```python
from build123d import *

# Parameters (mm, degrees)
SKETCH1_R           = 76
SKETCH1_R_2         = 27.051
SKETCH1_R_3         = 6.25
BOSS_EXTRUDE1_DEPTH = 7
SKETCH3_R           = 27.051
BOSS_EXTRUDE2_DEPTH = 5
SKETCH4_R           = 6.25
CUT_EXTRUDE1_DEPTH  = 10
FILLET1_R           = 5


with BuildPart() as part:
    # Sketch1 → Boss-Extrude1 (new body)
    with BuildSketch(Plane(origin=(0, 0, 0), x_dir=(1, 0, 0), z_dir=(0, 1, 0))):
        with Locations(Location((0, 0, 0), (0, 0, 270))):
            Circle(SKETCH1_R)
        with Locations(Location((0, 0, 0), (0, 0, 270))):
            Circle(SKETCH1_R_2, mode=Mode.SUBTRACT)
        with Locations(Location((0, 62.5, 0), (0, 0, 270))):
            Circle(SKETCH1_R_3, mode=Mode.SUBTRACT)
        with Locations(Location((62.5, 0, 0), (0, 0, 270))):
            Circle(SKETCH1_R_3, mode=Mode.SUBTRACT)
        with Locations(Location((0, -62.5, 0), (0, 0, 270))):
            Circle(SKETCH1_R_3, mode=Mode.SUBTRACT)
        with Locations(Location((-62.5, 0, 0), (0, 0, 270))):
            Circle(SKETCH1_R_3, mode=Mode.SUBTRACT)
    extrude(amount=BOSS_EXTRUDE1_DEPTH)

    # Sketch3 → Boss-Extrude2 (add)
    with BuildSketch(Plane.XZ):
        with Locations(Location((0, 0, 0), (0, 0, 270))):
            Circle(SKETCH3_R)
    extrude(amount=-BOSS_EXTRUDE2_DEPTH)

    # Sketch4 → Cut-Extrude1 (cut)
    with BuildSketch(Plane(origin=(0, 7, 0), x_dir=(1, 0, 0), z_dir=(0, 1, 0))):
        with BuildLine():
            Line((27.751246841, -43.661149418), (17.007161012, -32.917063589))
            ThreePointArc((17.007161012, -32.917063589), (15.274204293, -33.756114768), (13.5, -34.504008477))
            Line((13.5, -34.504008477), (13.5, -62.5))
            ThreePointArc((13.5, -62.5), (25.524772494, -58.625813335), (36.553123822, -52.463026398))
            Line((36.553123822, -52.463026398), (27.751246841, -43.661149418))
        make_face()
        with BuildLine():
            Line((62.5, -13.5), (34.504008477, -13.5))
            ThreePointArc((34.504008477, -13.5), (33.756114768, -15.274204293), (32.917063589, -17.007161012))
            Line((32.917063589, -17.007161012), (43.66114941, -27.751246833))
            Line((43.66114941, -27.751246833), (52.463026398, -36.553123822))
            ThreePointArc((52.463026398, -36.553123822), (58.625813335, -25.524772494), (62.5, -13.5))
        make_face()
        with BuildLine():
            ThreePointArc((-13.5, -34.504008477), (-15.274204293, -33.756114768), (-17.007161012, -32.917063589))
            Line((-17.007161012, -32.917063589), (-27.751246874, -43.66114945))
            Line((-27.751246874, -43.66114945), (-36.553123822, -52.463026398))
            ThreePointArc((-36.553123822, -52.463026398), (-25.524772494, -58.625813335), (-13.5, -62.5))
            Line((-13.5, -62.5), (-13.5, -34.504008477))
        make_face()
        with BuildLine():
            ThreePointArc((-32.917063589, -17.007161012), (-33.756114768, -15.274204293), (-34.504008477, -13.5))
            Line((-34.504008477, -13.5), (-62.5, -13.5))
            ThreePointArc((-62.5, -13.5), (-58.625813335, -25.524772494), (-52.463026398, -36.553123822))
            Line((-52.463026398, -36.553123822), (-43.661149471, -27.751246894))
            Line((-43.661149471, -27.751246894), (-32.917063589, -17.007161012))
        make_face()
        with BuildLine():
            ThreePointArc((-34.504008477, 13.5), (-33.756114768, 15.274204293), (-32.917063589, 17.007161012))
            Line((-32.917063589, 17.007161012), (-43.66114943, 27.751246854))
            Line((-43.66114943, 27.751246854), (-52.463026398, 36.553123822))
            ThreePointArc((-52.463026398, 36.553123822), (-58.625813335, 25.524772494), (-62.5, 13.5))
            Line((-62.5, 13.5), (-34.504008477, 13.5))
        make_face()
        with BuildLine():
            ThreePointArc((-17.007161012, 32.917063589), (-15.274204293, 33.756114768), (-13.5, 34.504008477))
            Line((-13.5, 34.504008477), (-13.5, 62.5))
            ThreePointArc((-13.5, 62.5), (-25.524772494, 58.625813335), (-36.553123822, 52.463026398))
            Line((-36.553123822, 52.463026398), (-27.751246874, 43.66114945))
            Line((-27.751246874, 43.66114945), (-17.007161012, 32.917063589))
        make_face()
        with BuildLine():
            ThreePointArc((36.553123822, 52.463026398), (25.524772494, 58.625813335), (13.5, 62.5))
            Line((13.5, 62.5), (13.5, 34.504008477))
            ThreePointArc((13.5, 34.504008477), (15.274204293, 33.756114768), (17.007161012, 32.917063589))
            Line((17.007161012, 32.917063589), (27.751246906, 43.661149483))
            Line((27.751246906, 43.661149483), (36.553123822, 52.463026398))
        make_face()
        with BuildLine():
            ThreePointArc((62.5, 13.5), (58.625813335, 25.524772494), (52.463026398, 36.553123822))
            Line((52.463026398, 36.553123822), (43.66114945, 27.751246874))
            Line((43.66114945, 27.751246874), (32.917063589, 17.007161012))
            ThreePointArc((32.917063589, 17.007161012), (33.756114768, 15.274204293), (34.504008477, 13.5))
            Line((34.504008477, 13.5), (62.5, 13.5))
        make_face()
        with Locations(Location((35.706198162, 35.706198162, 0), (0, 0, 270))):
            Circle(SKETCH4_R)
        with Locations(Location((35.706198162, -35.706198162, 0), (0, 0, 270))):
            Circle(SKETCH4_R)
        with Locations(Location((-35.706198162, -35.706198162, 0), (0, 0, 270))):
            Circle(SKETCH4_R)
        with Locations(Location((-35.706198162, 35.706198162, 0), (0, 0, 270))):
            Circle(SKETCH4_R)
    extrude(amount=-CUT_EXTRUDE1_DEPTH, mode=Mode.SUBTRACT)

    # Fillet1
    # the kernel refuses this fillet: 5 mm, written as the material it adds along each edge
    with BuildSketch(Plane(origin=(34.504008477, 7, 13.5), x_dir=(1, 0, 0), z_dir=(0, -1, 0)), Plane(origin=(13.5, 7, -34.504008477), x_dir=(0, 0, -1), z_dir=(0, -1, 0)), Plane(origin=(-34.504008477, 7, -13.5), x_dir=(-1, 0, 0), z_dir=(0, -1, 0)), Plane(origin=(-13.5, 7, 34.504008477), x_dir=(0, 0, 1), z_dir=(0, -1, 0))) as fillet1_piece_1:
        with BuildLine():
            CenterArc((3.258891319, 5), FILLET1_R, 206.100178987, 63.899821013)
            ThreePointArc((-1.231239688, 2.800290124), (-0.586707725, 1.412857227), (0, 0))
            Line((0, 0), (3.258891319, 0))
        make_face()
    extrude(amount=7)
    with BuildSketch(Plane(origin=(62.5, 7, 13.5), x_dir=(-1, 0, 0), z_dir=(0, -1, 0))) as fillet1_piece_2:
        with BuildLine():
            CenterArc((6.537189081, -5), FILLET1_R, 90, 108.2926811)
            ThreePointArc((1.789861186, -6.569355874), (0.807426008, -3.308519097), (0, 0))
            Line((0, 0), (6.537189081, 0))
        make_face()
    extrude(amount=7)
    with BuildSketch(Plane(origin=(52.463026398, 7, 36.553123822), x_dir=(-0.7071067811865521, 0, -0.707106781186543), z_dir=(0, -1, 0)), Plane(origin=(-36.553123822, 7, 52.463026398), x_dir=(0.7071067811865515, 0, -0.7071067811865436), z_dir=(0, -1, 0))) as fillet1_piece_3:
        with BuildLine():
            CenterArc((6.286852353, 5), FILLET1_R, 163.996405934, 106.003594066)
            ThreePointArc((1.480630334, 6.378488268), (0.658610883, 3.208210045), (0, 0))
            Line((0, 0), (6.286852353, 0))
        make_face()
    extrude(amount=7)
    with BuildSketch(Plane(origin=(32.917063589, 7, 17.007161012), x_dir=(0.4193809358930841, 0, -0.907810349472532), z_dir=(0, -1, 0)), Plane(origin=(17.007161012, 7, -32.917063589), x_dir=(-0.9078103494725283, 0, -0.41938093589309267), z_dir=(0, -1, 0)), Plane(origin=(-32.917063589, 7, -17.007161012), x_dir=(-0.4193809358930852, 0, 0.9078103494725317), z_dir=(0, -1, 0))) as fillet1_piece_4:
        with BuildLine():
            CenterArc((3.489548398, 4.995132399), FILLET1_R, 200.204490443, 67.267112024)
            Line((-1.202781391, 3.268273647), (0, 0))
            ThreePointArc((0, 0), (1.634487847, 0.036069898), (3.268975694, 0))
        make_face()
    extrude(amount=7)
    with BuildSketch(Plane(origin=(32.917063589, 7, -17.007161012), x_dir=(0.7071067811865526, 0, -0.7071067811865425), z_dir=(0, -1, 0)), Plane(origin=(-17.007161012, 7, -32.917063589), x_dir=(-0.7071067811865506, 0, -0.7071067811865445), z_dir=(0, -1, 0)), Plane(origin=(-32.917063589, 7, 17.007161012), x_dir=(-0.7071067811865506, 0, 0.7071067811865445), z_dir=(0, -1, 0)), Plane(origin=(17.007161012, 7, 32.917063589), x_dir=(0.7071067811865501, 0, 0.707106781186545), z_dir=(0, -1, 0))) as fillet1_piece_5:
        with BuildLine():
            CenterArc((3.482570273, 5), FILLET1_R, 202.732887976, 67.267112024)
            ThreePointArc((-1.129011858, 3.067822406), (-0.530655558, 1.546368727), (0, 0))
            Line((0, 0), (3.482570273, 0))
        make_face()
    extrude(amount=7)
    with BuildSketch(Plane(origin=(34.504008477, 7, -13.5), x_dir=(1, 0, 0), z_dir=(0, -1, 0))) as fillet1_piece_6:
        with BuildLine():
            CenterArc((3.258891319, -5), FILLET1_R, 90, 63.899821013)
            ThreePointArc((-1.231239688, -2.800290124), (-0.586707725, -1.412857227), (0, 0))
            Line((0, 0), (3.258891319, 0))
        make_face()
    extrude(amount=7)
    with BuildSketch(Plane(origin=(62.5, 7, -13.5), x_dir=(-1, 0, 0), z_dir=(0, -1, 0)), Plane(origin=(-13.5, 7, -62.5), x_dir=(0, 0, 1), z_dir=(0, -1, 0)), Plane(origin=(-62.5, 7, 13.5), x_dir=(1, 0, 0), z_dir=(0, -1, 0)), Plane(origin=(13.5, 7, 62.5), x_dir=(0, 0, -1), z_dir=(0, -1, 0))) as fillet1_piece_7:
        with BuildLine():
            CenterArc((6.537189081, 5), FILLET1_R, 161.7073189, 108.2926811)
            ThreePointArc((1.789861186, 6.569355874), (0.807426008, 3.308519097), (0, 0))
            Line((0, 0), (6.537189081, 0))
        make_face()
    extrude(amount=7)
    with BuildSketch(Plane(origin=(52.463026398, 7, -36.553123822), x_dir=(0.5289042688396526, 0, 0.848681491728901), z_dir=(0, -1, 0))) as fillet1_piece_8:
        with BuildLine():
            CenterArc((6.292063112, 4.993441128), FILLET1_R, 166.931450544, 106.003594066)
            Line((1.421561948, 6.124024341), (0, 0))
            ThreePointArc((0, 0), (3.274041034, -0.08387667), (6.548082068, 0))
        make_face()
    extrude(amount=7)
    with BuildSketch(Plane(origin=(36.553123822, 7, -52.463026398), x_dir=(-0.8486814917288963, 0, -0.52890426883966), z_dir=(0, -1, 0)), Plane(origin=(-52.463026398, 7, -36.553123822), x_dir=(-0.5289042688396536, 0, 0.8486814917289003), z_dir=(0, -1, 0))) as fillet1_piece_9:
        with BuildLine():
            CenterArc((6.292063112, -4.993441128), FILLET1_R, 87.06495539, 106.003594066)
            Line((1.421561948, -6.124024341), (0, 0))
            ThreePointArc((0, 0), (3.274041034, 0.08387667), (6.548082068, 0))
        make_face()
    extrude(amount=7)
    with BuildSketch(Plane(origin=(13.5, 7, -62.5), x_dir=(0.9648302017860143, 0, 0.26287388938720957), z_dir=(0, -1, 0)), Plane(origin=(-62.5, 7, -13.5), x_dir=(0.2628738893872084, 0, -0.9648302017860146), z_dir=(0, -1, 0)), Plane(origin=(-13.5, 7, 62.5), x_dir=(-0.9648302017860145, 0, -0.26287388938720885), z_dir=(0, -1, 0))) as fillet1_piece_10:
        with BuildLine():
            CenterArc((6.542607328, 4.992908013), FILLET1_R, 164.759342849, 108.2926811)
            Line((1.718456319, 6.30727746), (0, 0))
            ThreePointArc((0, 0), (3.404410363, -0.090694285), (6.808820725, 0))
        make_face()
    extrude(amount=7)
    with BuildSketch(Plane(origin=(-36.553123822, 7, -52.463026398), x_dir=(0.707106781186552, 0, 0.7071067811865429), z_dir=(0, -1, 0)), Plane(origin=(-52.463026398, 7, 36.553123822), x_dir=(0.7071067811865515, 0, -0.7071067811865436), z_dir=(0, -1, 0)), Plane(origin=(36.553123822, 7, 52.463026398), x_dir=(-0.7071067811865527, 0, -0.7071067811865425), z_dir=(0, -1, 0))) as fillet1_piece_11:
        with BuildLine():
            CenterArc((6.286852353, -5), FILLET1_R, 90, 106.003594066)
            ThreePointArc((1.480630334, -6.378488268), (0.658610883, -3.208210045), (0, 0))
            Line((0, 0), (6.286852353, 0))
        make_face()
    extrude(amount=7)
    with BuildSketch(Plane(origin=(-13.5, 7, -34.504008477), x_dir=(-0.9154220062230544, 0, 0.4024954043496127), z_dir=(0, -1, 0)), Plane(origin=(-34.504008477, 7, 13.5), x_dir=(0.4024954043496181, 0, 0.915422006223052), z_dir=(0, -1, 0)), Plane(origin=(13.5, 7, 34.504008477), x_dir=(0.915422006223051, 0, -0.40249540434962), z_dir=(0, -1, 0))) as fillet1_piece_12:
        with BuildLine():
            CenterArc((3.265421252, 4.995737851), FILLET1_R, 203.734271223, 63.899821013)
            Line((-1.311688779, 2.983260829), (0, 0))
            ThreePointArc((0, 0), (1.52950776, 0.031583378), (3.059015519, 0))
        make_face()
    extrude(amount=7)
    with BuildSketch(Plane(origin=(-17.007161012, 7, 32.917063589), x_dir=(-0.7071067811865496, 0, 0.7071067811865455), z_dir=(0, -1, 0))) as fillet1_piece_13:
        with BuildLine():
            CenterArc((3.482570273, -5), FILLET1_R, 90, 67.267112024)
            ThreePointArc((-1.129011858, -3.067822406), (-0.530655558, -1.546368727), (0, 0))
            Line((0, 0), (3.482570273, 0))
        make_face()
    extrude(amount=7)


solid = part.part
```
Check sheet for the modelled part. Datum: model origin and axes. Units: mm. A direction names the side the tool comes from. Coordinates: 2 decimals unless noted, no trailing zeros. Write each loop counter-clockwise with the first axis right and the second up, starting at its lowest first coordinate (ties: lowest second). Pieces come first, ordered by that corner, then holes. Notation, with made-up numbers: M -3,-31.5 L 44,-31.5 A21 ccw 44,-10.5 Z; hole C -10.75,-39.5 d3. An arc over 180 degrees is marked long. Write item = value, one per line. Start each with the question number.
1. Sectioned sample at A-A (x = 0). Record the cut outline in (y, z), then the cut area to 3 significant figures.
2. Thickness scan on probe 1 along X at (y, z) = (5.95, 0); probe 2 along X at (y, z) = (4.5, 0); probe 3 along X at (y, z) = (2.5, -30). Record the ranges inside material, lowest first.
3. Sectioned sample at C-C (y = 3.5). State how many separate pieces and enclosed holes the cut face has, then the cut area to 3 significant figures.
4. Tool access check on faces 3 (the cylindrical face through (52.185, 3.549, -33.532)), 4 (the flat face through (0, 5, 0)). Record the directions out of +Z, -Z, +X, -X, +Y, -Y that give a thin tool (end or side, any length) a straight path to the whole face; none if there is none.
5. Go/stop test with flat-tipped pins: pin 1 (3.5 mm diameter, centred on x = 46.5, y = 5, fed in from -Z); pin 2 (3 mm diameter, centred on y = 3.5, z = 34.5, fed in from +X); pin 3 (1 mm diameter, centred on x = 8.5, y = 4.5, fed in from -Z). Record where each tip stops, or that it passes through.
6. Mould release check, pull along Z, two halves, no side actions. Record for faces 1 (the flat face through (22, 7, -24)), 2 (the flat face through (-47, 4, -13.5)): pulls with the +Z half, pulls with the -Z half, needs draft (parallel to the pull), parting line crosses it, or undercut.
7. Sectioned sample at B-B (z = 0). Record the cut outline in (x, y).
The answers:
q1.outline = M 0,-76 L 7,-76 L 7,-68.75 L 0,-68.75 Z; M 0,-56.25 L 7,-56.25 L 7,-27.05 L 5,-27.05 L 5,27.05 L 7,27.05 L 7,56.25 L 0,56.25 Z; M 0,68.75 L 7,68.75 L 7,76 L 0,76 Z
q1.area = 781 mm²
q2.probe_1 = -76 to -68.75, -56.25 to -27.05, 27.05 to 56.25, 68.75 to 76
q2.probe_2 = -76 to -68.75, -56.25 to 56.25, 68.75 to 76
q2.probe_3 = -69.83 to -56.47, -45.91 to -38.26, -33.16 to 33.16, 38.26 to 45.91, 56.47 to 69.83
q3.separate_pieces = 1
q3.enclosed_holes = 16
q3.area = 14,200 mm²
q4.face_3 = +Y, -Y
q4.face_4 = +Y
q5.pin_1 = -61.43
q5.pin_2 = 68.46
q5.pin_3 = -75.58
q6.face_1 = needs draft
q6.face_2 = undercut
q7.outline = M -76,0 L -68.75,0 L -68.75,7 L -76,7 Z; M -56.25,0 L 56.25,0 L 56.25,7 L 27.05,7 L 27.05,5 L -27.05,5 L -27.05,7 L -56.25,7 Z; M 68.75,0 L 76,0 L 76,7 L 68.75,7 Z
